from build123d import *

# Parameters (mm, degrees)
F0_W     = 150
F0_H     = 50
F1_DEPTH = 10
F3_DEPTH = 10.001
F4_SIZE  = 2


with BuildPart() as f1:
    # F0 (on Front) → F1 (new body)
    with BuildSketch(Plane.XZ):
        Rectangle(F0_W, F0_H)
    extrude(amount=F1_DEPTH)

    # F2 (on face) → F3 (cut, through all)
    with BuildSketch(Plane.XZ.offset(10)):
        with BuildLine():
            ThreePointArc((-28, -5), (-30, -3), (-32, -5))
            Line((-32, -5), (-28, -5))
        make_face()
        with BuildLine():
            Line((-28, -5), (-32, -5))
            ThreePointArc((-32, -5), (-30, -7), (-28, -5))
        make_face()
        with BuildLine():
            ThreePointArc((-58, -5), (-60, -3), (-62, -5))
            Line((-62, -5), (-58, -5))
        make_face()
        with BuildLine():
            Line((-58, -5), (-62, -5))
            ThreePointArc((-62, -5), (-60, -7), (-58, -5))
        make_face()
        with BuildLine():
            ThreePointArc((32, -5), (30, -3), (28, -5))
            Line((28, -5), (32, -5))
        make_face()
        with BuildLine():
            Line((32, -5), (28, -5))
            ThreePointArc((28, -5), (30, -7), (32, -5))
        make_face()
        with BuildLine():
            Line((58, -5), (62, -5))
            ThreePointArc((62, -5), (60, -3), (58, -5))
        make_face()
        with BuildLine():
            ThreePointArc((58, -5), (60, -7), (62, -5))
            Line((62, -5), (58, -5))
        make_face()
    extrude(amount=-F3_DEPTH, mode=Mode.SUBTRACT)

    # F4
    f4_edges = [f1.edges().sort_by_distance(p)[0] for p in [
        (-58, -10, -5),
        (-28, -10, -5),
        (32, -10, -5),
        (62, -10, -5),
    ]]
    chamfer(f4_edges, length=F4_SIZE)


solid = f1.part
Here's how the part is built. I have some questions about the finished solid (model axes, mm). Coordinates: 2 decimals unless noted, no trailing zeros. Order: outer loops, then holes, each group sorted by start corner. A loop starts at its lowest first (then second) coordinate and runs counter-clockwise, first axis right, second up. Notation, with made-up numbers: M 81.25,1 L 93.25,1 A22 cw 93.25,12 Z; hole C 70,33.5 d5. An arc over 180 degrees is marked long. Answer as CSV lines item,"result".
Item 1: If I drill on line 1 (X direction, y = -4, z = -5); line 2 (Z direction, x = 30, y = -5.25), over which ranges is the centre line in solid material (lowest first)?
Results found:
line 1,"-75 to -62, -58 to -32, -28 to 28, 32 to 58, 62 to 75"
line 2,"-25 to -7, -3 to 25"
Item 2: We'd pull the mould along Z, two halves only. Please class faces 1 (the face through (-75, -5, 0)), 2 (the face through (-58, -4, -5)), 3 (the face through (-1, -5, -25)), 4 (the face through (-1, -5, 25)): +Z half, -Z half, draft (parallel to the pull), parting line (faces both ways), or undercut.
Results found:
face 1,"draft"
face 2,"undercut"
face 3,"-Z half"
face 4,"+Z half"
Item 3: Imagine slicing it at A-A on x = 30. Write out the boundary of the cut face in (y, z), plus the area to 3 significant figures.
Results found:
outline,"M -10,-25 L 0,-25 L 0,-7 L -8,-7 L -10,-9 Z; M -10,-1 L -8,-3 L 0,-3 L 0,25 L -10,25 Z"
area,"456 mm2"
Item 4: Imagine slicing it at B-B on z = -5. Write out the boundary of the cut face in (x, y).
Results found:
outline,"M -75,-10 L -64,-10 L -62,-8 L -62,0 L -75,0 Z; M -58,-8 L -56,-10 L -34,-10 L -32,-8 L -32,0 L -58,0 Z; M -28,-8 L -26,-10 L 26,-10 L 28,-8 L 28,0 L -28,0 Z; M 32,-8 L 34,-10 L 56,-10 L 58,-8 L 58,0 L 32,0 Z; M 62,-8 L 64,-10 L 75,-10 L 75,0 L 62,0 Z"
